```python
from build123d import *

# Parameters (mm, degrees)
CHAMFER_1_SIZE         = 0.8
CHAMFER_1_SIZE2        = 0.461880215
CHAMFER_1_PART_2_SIZE  = 0.8
CHAMFER_1_PART_2_SIZE2 = 0.461880215


with BuildPart() as part:
    # Эскиз1 → Повернуть1 (revolve)
    with BuildSketch(Plane(origin=(0, 0, 0), x_dir=(0, 0, -1), z_dir=(1, 0, 0))):
        Polygon((0, 13), (36, 13), (36, 14.5), (18.854921546, 16), (16, 16), (16, 18), (7, 18), (7, 16), (4, 16), (4, 24.5), (0, 24.5), align=None)
    revolve(axis=Axis((0, 0, 0), (0, 0, -1)))

    # Фаска1
    chamfer_1_edges = [part.edges().sort_by_distance(p)[0] for p in [
        (0, -18, -7),
    ]]
    chamfer_1_side = [part.faces().sort_by_distance(p)[0] for p in [
        (0, -17.490883118, -7),
    ]]
    chamfer(chamfer_1_edges, length=CHAMFER_1_SIZE, length2=CHAMFER_1_SIZE2, reference=chamfer_1_side[0])

    # Фаска1 part 2
    chamfer_1_part_2_edges = [part.edges().sort_by_distance(p)[0] for p in [
        (0, -18, -16),
    ]]
    chamfer_1_part_2_side = [part.faces().sort_by_distance(p)[0] for p in [
        (0, -16.509116882, -16),
    ]]
    chamfer(chamfer_1_part_2_edges, length=CHAMFER_1_PART_2_SIZE, length2=CHAMFER_1_PART_2_SIZE2, reference=chamfer_1_part_2_side[0])


solid = part.part
```
The model under review builds one solid part; all positions refer to its coordinate system, in mm. A direction names the side the tool comes from. Coordinates: 2 decimals unless noted, no trailing zeros. Write each loop counter-clockwise with the first axis right and the second up, starting at its lowest first coordinate (ties: lowest second). Pieces come first, ordered by that corner, then holes. Notation, with made-up numbers: (-16.5, 87.5) - (-1.5, 87.5) arc R19 cw to (-1.5, 114.5) - close; hole circle Ø11 at (32, -23). An arc over 180 degrees is marked (long way). Answer in a Markdown table with one row per item. Add a question column.
Q1. Draft analysis for pull direction Z (two halves, no side actions). For faces 1 (the face through (4.53, 14.4, -29.21)), 2 (the face through (-15.62, -3.47, -5.48)), 3 (the face through (-5, -16, -4)), 4 (the face through (20.66, 13.17, -1.97)), state which applies: +Z half, -Z half, draft (parallel to the pull), parting line (faces both ways), or undercut.
Q2. For faces 5 (the face through (-13, -10, -16)), 6 (the face through (-13, 10, -7)), 7 (the face through (10, 9, -36)), list the 3-axis set-ups (+Z, -Z, +X, -X, +Y, -Y) from which the entire face can be reached by the end or side of a thin tool; tool diameter is ignored.
Q3. To check wall thickness, follow line 1 along Z through (x, y) = (-16, 3); line 2 along Y through (x, z) = (-3, -14.5); line 3 along Z through (x, y) = (19, 1.5). State the ranges of each line that lie inside material, in increasing order. Write a range as from..to.
Q4. Consider section C-C on z = -10.5. Give the boundary of the cut face in (x, y).
Q5. Consider section D-D on z = -31. Give the boundary of the cut face in (x, y), then the cut area to 3 significant figures.
Q6. Clearance check with flat-ended pins moving along their axes: pin 1 (5 mm diameter, centred on x = -8, z = -20, fed in from -Y); pin 2 (12 mm diameter, centred on y = 10, z = -30, fed in from +X); pin 3 (4 mm diameter, centred on y = 4.5, z = -9, fed in from +X). State where each tip first meets the part, or that it passes through.
Q7. Consider section A-A on y = 0. Give the boundary of the cut face in (x, z).
Answers below:
| question | item | result |
|---|---|---|
| 1 | face 1 | -Z half |
| 1 | face 2 | undercut |
| 1 | face 3 | undercut |
| 1 | face 4 | draft |
| 2 | face 5 | -Z |
| 2 | face 6 | none |
| 2 | face 7 | -Z, +X, -X, +Y, -Y |
| 3 | line 1 | -16..-7, -4..0 |
| 3 | line 2 | -17.75..-12.65, 12.65..17.75 |
| 3 | line 3 | -4..0 |
| 4 | outline | circle Ø36 at (0, 0); hole circle Ø26 at (0, 0) |
| 5 | outline | circle Ø29.87 at (0, 0); hole circle Ø26 at (0, 0) |
| 5 | area | 170 mm² |
| 6 | pin 1 | y = -14.95 |
| 6 | pin 2 | x = 14.57 |
| 6 | pin 3 | x = 17.83 |
| 7 | outline | (-24.5, -4) - (-16, -4) - (-16, -7) - (-17.2, -7) - (-18, -7.46) - (-18, -15.54) - (-17.2, -16) - (-16, -16) - (-16, -18.85) - (-14.5, -36) - (-13, -36) - (-13, 0) - (-24.5, 0) - close; (13, -36) - (14.5, -36) - (16, -18.85) - (16, -16) - (17.2, -16) - (18, -15.54) - (18, -7.46) - (17.2, -7) - (16, -7) - (16, -4) - (24.5, -4) - (24.5, 0) - (13, 0) - close |
